Can you work these out from the model? Positions are in its coordinate system, mm. A direction names the side the tool comes from. Round coordinates to 2 decimals unless told otherwise and drop trailing zeros. Loops run counter-clockwise (first coordinate to the right, second up) from the corner with the lowest first, then second, coordinate; pieces in that order, holes last. Notation, with made-up numbers: (-35, 86.5) -> (-15, 86.5) arc R30 ccw to (-15, 124.5) -> close; hole circle Ø6 at (78, 65). An arc over 180 degrees is marked (long way). Write each question's results on one line, items separated by ' | '.
from build123d import *

# Parameters (mm, degrees)
SKETCH1_W               = 1000
SKETCH1_H               = 80
BOSS_EXTRUDE1_DEPTH     = 65
FILLET1_R               = 2.5
CUT_EXTRUDE1_DEPTH      = 993.937560978
CUT_EXTRUDE1_DEPTH_BACK = 65


with BuildPart() as part:
    # Sketch1 → Boss-Extrude1 (new body)
    with BuildSketch(Plane(origin=(0, 0, 0), x_dir=(1, 0, 0), z_dir=(0, 1, 0))):
        with Locations((490, 0)):
            Rectangle(SKETCH1_W, SKETCH1_H)
    extrude(amount=-BOSS_EXTRUDE1_DEPTH)

    # Fillet1
    fillet1_edges = [part.edges().sort_by_distance(p)[0] for p in [
        (490, 0, 40),
        (490, 0, -40),
    ]]
    fillet(fillet1_edges, radius=FILLET1_R)

    # Sketch2 → Cut-Extrude1 (cut, two sides: drawn at the far end of the back side and taken through both)
    with BuildSketch(Plane(origin=(0, 0, 0), x_dir=(0, 0, -1), z_dir=(1, 0, 0)).offset(-CUT_EXTRUDE1_DEPTH_BACK)):
        with BuildLine():
            Line((39.2, -64.2), (39.2, -67.2))
            Line((39.2, -67.2), (-39.2, -67.2))
            Line((-39.2, -67.2), (-39.2, -64.2))
            Line((-39.2, -64.2), (-39.2, -2.5))
            ThreePointArc((-39.2, -2.5), (-38.702081528, -1.297918472), (-37.5, -0.8))
            Line((-37.5, -0.8), (37.5, -0.8))
            ThreePointArc((37.5, -0.8), (38.702081528, -1.297918472), (39.2, -2.5))
            Line((39.2, -2.5), (39.2, -64.2))
        make_face()
    extrude(amount=CUT_EXTRUDE1_DEPTH + CUT_EXTRUDE1_DEPTH_BACK, mode=Mode.SUBTRACT)


solid = part.part
1. If we section it at B-B (x = 322): List the corners of the cut face in (y, z) for me, then the cut area to 3 significant figures.
Final values:
outline: (-65, -40) -> (-2.5, -40) arc R2.5 ccw to (0, -37.5) -> (0, 37.5) arc R2.5 ccw to (-2.5, 40) -> (-65, 40) -> (-65, 39.2) -> (-2.5, 39.2) arc R1.7 cw to (-0.8, 37.5) -> (-0.8, -37.5) arc R1.7 cw to (-2.5, -39.2) -> (-65, -39.2) -> close | area: 165 mm2
2. Will this pin go through, and if not, where does the flat tip stop? pin 1 (8 mm diameter, centred on x = 442, z = 8, fed in from -Y).
Final values:
pin 1: y = -0.8
3. On a 3-axis mill with a long thin cutter (end or side, diameter ignored), from which of +Z, -Z, +X, -X, +Y, -Y can I reach the whole of each face in a straight line? I mean faces 1 (the face through (483, -33, -39.2)), 2 (the face through (483, -33, -40)). Say none if no direction works.
Final values:
face 1: +X, -X, -Y | face 2: -Z, +X, -X, +Y, -Y
4. We'd pull the mould along Z, two halves only. Please class faces 3 (the face through (483, -33, 40)), 4 (the face through (483, 0, -1)), 5 (the face through (483, -0.8, 1)), 6 (the face through (483, -34, 39.2)): pulls with the +Z half, pulls with the -Z half, needs draft (parallel to the pull), parting line crosses it, or undercut.
Final values:
face 3: pulls with the +Z half | face 4: needs draft | face 5: undercut | face 6: undercut
5. If we section it at C-C (z = 29): List the corners of the cut face in (x, y) for me.
Final values:
outline: (-10, -0.8) -> (990, -0.8) -> (990, 0) -> (-10, 0) -> close
6. If we section it at A-A (y = -22): List the corners of the cut face in (x, z) for me.
Final values:
outline: (-10, -40) -> (990, -40) -> (990, -39.2) -> (-10, -39.2) -> close; (-10, 39.2) -> (990, 39.2) -> (990, 40) -> (-10, 40) -> close
7. Please list where these lines run through material, in increasing order: line 1 (Z direction, x = 441.5, y = -44); line 2 (Y direction, x = 186, z = 7). Write a range as from..to.
Final values:
line 1: -40..-39.2, 39.2..40 | line 2: -0.8..0
